from build123d import *

# Parameters (mm, degrees)
BOSS_EXTRUDE1_DEPTH            = 20
CBORE_FOR_M4_SHCS1_D           = 4.7
CBORE_FOR_M4_SHCS1_CBORE_D     = 8
CBORE_FOR_M4_SHCS1_CBORE_DEPTH = 4
FILLET1_R                      = 1
FILLET1_OF_MIRROR1_R           = 1


with BuildPart() as part:
    # Sketch1 → Boss-Extrude1 (new body)
    with BuildSketch(Plane.XY):
        with BuildLine():
            Line((0, 0), (0, 9))
            ThreePointArc((0, 9), (0.292893219, 9.707106781), (1, 10))
            Line((1, 10), (14, 10))
            ThreePointArc((14, 10), (14.707106781, 10.292893219), (15, 11))
            Line((15, 11), (15, 29))
            ThreePointArc((15, 29), (15.292893219, 29.707106781), (16, 30))
            Line((16, 30), (65, 30))
            Line((65, 30), (65, 20))
            Line((65, 20), (25, 20))
            Line((25, 20), (25, 0))
            Line((25, 0), (0, 0))
        make_face()
    boss_extrude1 = extrude(amount=BOSS_EXTRUDE1_DEPTH)

    # CBORE for M4 SHCS1 (through all)
    with Locations(Plane(origin=(0, 10, 0), x_dir=(1, 0, 0), z_dir=(0, 1, 0))):
        with Locations((7.5, -10)):
            cbore_for_m4_shcs1 = CounterBoreHole(CBORE_FOR_M4_SHCS1_D / 2, CBORE_FOR_M4_SHCS1_CBORE_D / 2, CBORE_FOR_M4_SHCS1_CBORE_DEPTH)

    # Fillet1
    fillet1_edges = [part.edges().sort_by_distance(p)[0] for p in [
        (45, 20, 20),
        (0, 4.5, 0),
        (0.292893219, 9.707106781, 0),
        (7.5, 10, 0),
        (14.707106781, 10.292893219, 0),
        (15, 20, 0),
        (15.292893219, 29.707106781, 0),
        (40.5, 30, 0),
        (45, 20, 0),
        (25, 10, 0),
        (40.5, 30, 20),
        (15.292893219, 29.707106781, 20),
        (15, 20, 20),
        (14.707106781, 10.292893219, 20),
        (7.5, 10, 20),
        (0.292893219, 9.707106781, 20),
        (0, 4.5, 20),
        (25, 10, 20),
    ]]
    fillet(fillet1_edges, radius=FILLET1_R)

    # Mirror1: Boss-Extrude1, CBORE for M4 SHCS1 across plane
    add(boss_extrude1.mirror(Plane(origin=(65, 30, 20), x_dir=(0, 0, 1), z_dir=(-1, 0, 0))))
    add(cbore_for_m4_shcs1.mirror(Plane(origin=(65, 30, 20), x_dir=(0, 0, 1), z_dir=(-1, 0, 0))), mode=Mode.SUBTRACT)

    # Fillet1 of Mirror1
    fillet1_of_mirror1_edges = [part.edges().sort_by_distance(p)[0] for p in [
        (85, 20, 20),
        (130, 4.5, 0),
        (129.707106781, 9.707106781, 0),
        (122.5, 10, 0),
        (115.292893219, 10.292893219, 0),
        (115, 20, 0),
        (114.707106781, 29.707106781, 0),
        (89.5, 30, 0),
        (85, 20, 0),
        (105, 10, 0),
        (89.5, 30, 20),
        (114.707106781, 29.707106781, 20),
        (115, 20, 20),
        (115.292893219, 10.292893219, 20),
        (122.5, 10, 20),
        (129.707106781, 9.707106781, 20),
        (130, 4.5, 20),
        (105, 10, 20),
    ]]
    fillet(fillet1_of_mirror1_edges, radius=FILLET1_OF_MIRROR1_R)


solid = part.part
Work out the finished part from the listing and answer in its coordinate system (mm). A direction names the side the tool comes from. Round coordinates to 2 decimals unless told otherwise and drop trailing zeros. Loops run counter-clockwise (first coordinate to the right, second up) from the corner with the lowest first, then second, coordinate; pieces in that order, holes last. Notation, with made-up numbers: (-27, -35) - (13, -35) arc R26 ccw to (13, -8) - close; hole circle Ø7 at (-10.75, -9). An arc over 180 degrees is marked (long way). Use one line per item in the form item = value. Start each with the question number.
(1) Find section D-D on z = 16.5. Determine the outline of the cut face in (x, y).
(2) Find section C-C on y = 18.5. Determine the outline of the cut face in (x, z).
(3) Find section B-B on x = 7.5. Determine the outline of the cut face in (y, z), and give its area (3 significant figures).
(4) Consider line 1 (X direction, y = 4.6, z = 10); line 2 (Z direction, x = 122.5, y = 6.95); line 3 (Z direction, x = 122.5, y = 2.5). Determine where each line is inside the solid, lowest interval first.
(5) Which of the six approach directions +Z, -Z, +X, -X, +Y, -Y give full straight-line access (tool end or side, diameter ignored) to faces 1 (the face through (9, 10, 6)), 2 (the face through (121, 6, 12)), 3 (the face through (25, 10, 10))?
(6) Flat-ended cylindrical pins translate along their axes: P1, Ø0.5, axis at y = 29.5, z = 0.5, coming from the -X side; P2, Ø5, axis at x = 7.5, z = 10, coming from the +Y side; P3, Ø5.5, axis at y = 18, z = 8, coming from the +X side. Find the tip coordinate at first contact, or state that the pin passes through.
(7) Find section A-A on z = 10. Give the number of separate pieces and of enclosed holes in the cut face, and give its area (3 significant figures).
(8) Determine the mould class of faces 4 (the face through (9, 6, 12)), 5 (the face through (15, 20, 10)), 6 (the face through (64, 24, 0)), 7 (the face through (8.009, 2.958, 12.294)) for opening direction Z: +Z half, -Z half, draft (parallel to the pull), parting line (faces both ways), or undercut.
Answer list:
q1.outline = (0, 0) - (25, 0) - (25, 20) - (105, 20) - (105, 0) - (130, 0) - (130, 9) arc R1 ccw to (129, 10) - (116, 10) arc R1 cw to (115, 11) - (115, 29) arc R1 ccw to (114, 30) - (16, 30) arc R1 ccw to (15, 29) - (15, 11) arc R1 cw to (14, 10) - (1, 10) arc R1 ccw to (0, 9) - close
q2.outline = (15, 1) arc R1 ccw to (16, 0) - (24, 0) arc R1 ccw to (25, 1) - (25, 19) arc R1 ccw to (24, 20) - (16, 20) arc R1 ccw to (15, 19) - close; (105, 1) arc R1 ccw to (106, 0) - (114, 0) arc R1 ccw to (115, 1) - (115, 19) arc R1 ccw to (114, 20) - (106, 20) arc R1 ccw to (105, 19) - close
q3.outline = (0, 0) - (9, 0) arc R1 ccw to (10, 1) - (10, 6) - (6, 6) - (6, 7.65) - (0, 7.65) - close; (0, 12.35) - (6, 12.35) - (6, 14) - (10, 14) - (10, 19) arc R1 ccw to (9, 20) - (0, 20) - close
q3.area = 139 mm^2
q4.line_1 = 0 to 5.15, 9.85 to 25, 105 to 120.15, 124.85 to 130
q4.line_2 = 0 to 6, 14 to 20
q4.line_3 = 0 to 7.65, 12.35 to 20
q5.face_1 = +Z, -Z, -X, +Y
q5.face_2 = +Y
q5.face_3 = +Z, -Z, -Y
q6.P1 = 15.11
q6.P2 = 6
q6.P3 = 115
q7.separate_pieces = 3
q7.enclosed_holes = 0
q7.area = 1,580 mm^2
q8.face_4 = undercut
q8.face_5 = draft
q8.face_6 = -Z half
q8.face_7 = undercut
